Read the model definition and answer for the solid it produces. Units are mm, in the model's axes. Face numbers are marked on the shaded views. A direction names the side the tool comes from. Coordinates: 2 decimals unless noted, no trailing zeros. Order: outer loops, then holes, each group sorted by start corner. A loop starts at its lowest first (then second) coordinate and runs counter-clockwise, first axis right, second up. Notation, with made-up numbers: (48, 31) -> (59, 31) arc R15 ccw to (59, 42) -> close; hole circle Ø8 at (55, -20.5). An arc over 180 degrees is marked (long way). Answer as a JSON object with one key per item and string values. Group by question number.
1) A tool of negligible diameter and unlimited length cuts with its end or side. For the marked faces 4, 5 and 6, from which of +Z, -Z, +X, -X, +Y, -Y can it reach the whole face along a straight path? Write none if from no direction.
2) Section A-A on y = 12.25 is taken. Determine the outline of the cut face in (x, z), and give its area (3 significant figures).
3) Section B-B on z = 3.5 is taken. Determine the outline of the cut face in (x, y), and give its area (3 significant figures).
4) Determine the mould class of the marked faces 1, 2 and 3 for opening direction X: released by +X, released by -X, zero draft, split by the parting line, or undercut.
5) Consider L1, parallel to X at y = 14, z = 2.5; L2, parallel to Z at x = 5.25, y = 6; L3, parallel to X at y = 16, z = 9.25. Determine where each line is inside the solid, lowest interval first.
6) Given pin 1 (2 mm diameter, centred on x = 3.5, y = 9.5, fed in from +Z); pin 2 (2 mm diameter, centred on y = 8, z = 10, fed in from -X); pin 3 (1 mm diameter, centred on y = 21.5, z = 3.5, fed in from -X), each flat-ended and moving along its own axis, determine where each tip first touches the part or whether it passes through.
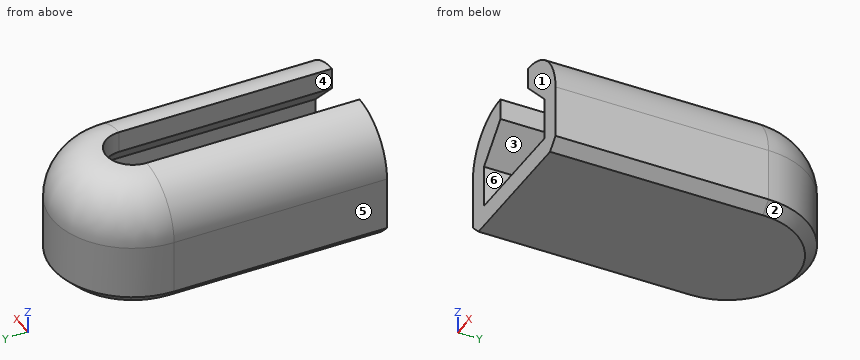
from build123d import *

# Parameters (mm, degrees)
F3_DEPTH = 2
F4_SIZE  = 1


with BuildPart() as f2:
    # F2: sweep along a path in F1
    with BuildLine(Plane.XY) as f2_path:
        Line((0, 0), (0, 20))
        ThreePointArc((0, 20), (2.1966991411, 25.3033008589), (7.5, 27.5))
        ThreePointArc((7.5, 27.5), (12.8033008589, 25.3033008589), (15, 20))
        Line((15, 20), (15, 0))
    # F0 (on Front) → F2 (sweep)
    with BuildSketch(Plane.XZ):
        with BuildLine():
            Line((0, 6), (0, 0))
            Line((0, 0), (2, 0))
            Line((2, 0), (2, 6.0000002682))
            Line((2, 6.0000002682), (5, 9.0000002682))
            Line((5, 9.0000002682), (5, 11))
            ThreePointArc((5, 11), (1.4644660941, 9.5355339059), (0, 6))
        make_face()
    sweep(path=f2_path.line)

    # F1 (on Top) → F3 (join)
    with BuildSketch(Plane.XY):
        with BuildLine():
            Line((0, 20), (0, 0))
            Line((0, 0), (7.5, 0))
            Line((7.5, 0), (15, 0))
            Line((15, 0), (15, 20))
            ThreePointArc((15, 20), (12.8033008589, 25.3033008589), (7.5, 27.5))
            ThreePointArc((7.5, 27.5), (2.1966991411, 25.3033008589), (0, 20))
        make_face()
    extrude(amount=F3_DEPTH)

    # F4
    f4_edges = [f2.edges().sort_by_distance(p)[0] for p in [
        (0, 10, 0),
        (7.5, 27.5, 0),
        (15, 10, 0),
    ]]
    chamfer(f4_edges, length=F4_SIZE)


solid = f2.part
Worked answers:
{
 "1": {"face 4": "+Z, -Y", "face 5": "+Z, -Z, -X, +Y, -Y", "face 6": "-Y"},
 "2": {"outline": "(0, 1) -> (1, 0) -> (14, 0) -> (15, 1) -> (15, 6) arc R5 ccw to (10, 11) -> (10, 9) -> (13, 6) -> (13, 2) -> (2, 2) -> (2, 6) -> (5, 9) -> (5, 11) arc R5 ccw to (0, 6) -> close", "area": "75.3 mm²"},
 "3": {"outline": "(0, 0) -> (2, 0) -> (2, 20) arc R5.5 cw to (13, 20) -> (13, 0) -> (15, 0) -> (15, 20) arc R7.5 ccw to (0, 20) -> close", "area": "121 mm²"},
 "4": {"face 1": "zero draft", "face 2": "split by the parting line", "face 3": "undercut"},
 "5": {"L1": "x = 0 to 2, 13 to 15", "L2": "z = 0 to 2", "L3": "x = 1.2 to 5, 10 to 13.8"},
 "6": {"pin 1": "stops at z = 10.97", "pin 2": "stops at x = 1", "pin 3": "stops at x = 0.07"}
}
